Input: part model. Units: mm. Frame: model coordinates. A direction names the side the tool comes from. Give positions to 0.01 mm unless a question says otherwise; leave off trailing zeros. Order: outer loops, then holes, each group sorted by start corner. A loop starts at its lowest first (then second) coordinate and runs counter-clockwise, first axis right, second up. Notation, with made-up numbers: (-3.75, 12.5) - (49.25, 12.5) arc R15 cw to (49.25, 38.5) - close; hole circle Ø1 at (-36, 73). An arc over 180 degrees is marked (long way). Use a Markdown table: item, result.
from build123d import *

# Parameters (mm, degrees)
PAD_DEPTH    = 35
POCKET_DEPTH = 30
SKETCH003_W  = 25
SKETCH003_H  = 15
PAD001_DEPTH = 2
FILLET_R     = 0.99
FILLET001_R  = 0.96
FILLET002_R  = 3


with BuildPart() as part:
    # Sketch → Pad (new body)
    with BuildSketch(Plane.XY):
        with BuildLine():
            ThreePointArc((20, 0), (0, 6.835898), (-20, 0))
            Line((-20, -5.3), (-20, 0))
            Line((20, -5.3), (-20, -5.3))
            Line((20, 0), (20, -5.3))
        make_face()
    extrude(amount=PAD_DEPTH)

    # Sketch002 → Pocket (cut)
    with BuildSketch(Plane(origin=(3, 0, 37), x_dir=(0.965926, 0, -0.258819), z_dir=(0.258819, 0, 0.965926))):
        Polygon((-5.6, -0.240433), (5.6, -0.240433), (5.6, -2.440433), (2.7, -5.340433), (-2.7, -5.340433), (-5.6, -2.440433), align=None)
    extrude(amount=-POCKET_DEPTH, mode=Mode.SUBTRACT)

    # Sketch003 (on Face4 of Pocket) → Pad001 (join)
    with BuildSketch(Plane(origin=(0, 0, 0), x_dir=(1, 0, 0), z_dir=(0, 0, -1))):
        with Locations((0, -10.470599)):
            Rectangle(SKETCH003_W, SKETCH003_H)
    extrude(amount=-PAD001_DEPTH)

    # Fillet
    fillet_edges = [part.edges().sort_by_distance(p)[0] for p in [
        (-12.5, 11.160507, 2),
        (0, 17.970599, 2),
        (12.5, 11.160507, 2),
        (-12.5, 11.160507, 0),
        (0, 17.970599, 0),
        (12.5, 11.160507, 0),
    ]]
    fillet(fillet_edges, radius=FILLET_R)

    # Fillet001
    fillet001_edges = [part.edges().sort_by_distance(p)[0] for p in [
        (-12.149588, 17.620187, 1.765663),
        (-12.149588, 17.620187, 0.234337),
        (12.149588, 17.620187, 0.234337),
        (12.149588, 17.620187, 1.765663),
    ]]
    fillet(fillet001_edges, radius=FILLET001_R)

    # Fillet002
    fillet002_edges = [part.edges().sort_by_distance(p)[0] for p in [
        (-20, 0, 17.5),
        (20, 0, 17.5),
    ]]
    fillet(fillet002_edges, radius=FILLET002_R)


solid = part.part
1. Pin query (flat end, axial travel): pin 1 (2 mm diameter, centred on x = 4, y = 11.5, fed in from +Z); pin 2 (8 mm diameter, centred on y = 4, z = 19.5, fed in from +X); pin 3 (10 mm diameter, centred on y = 5, z = 21.5, fed in from -X); pin 4 (1.5 mm diameter, centred on y = -1, z = 3.5, fed in from +X). Return the tip coordinate at first contact, or that it passes through.
Response:
| item | result |
|---|---|
| pin 1 | stops at z = 2 |
| pin 2 | stops at x = 19.59 |
| pin 3 | stops at x = -19.59 |
| pin 4 | stops at x = 20 |
2. Material intervals for line 1 along Z through (x, y) = (6, 8.5); line 2 along Y through (x, z) = (1.5, 14); line 3 along Y through (x, z) = (-0.5, 9), sorted ascending.
Response:
| item | result |
|---|---|
| line 1 | z = 0 to 2 |
| line 2 | y = -5.3 to -3.54, -0.24 to 6.8 |
| line 3 | y = -5.3 to -4.17, -0.24 to 6.83 |
3. Set-up query: faces 1 (the face through (-12.22, 10.59, 0.3)), 2 (the face through (-4.689, -2.735, 8.002)), 3 (the face through (12.2, 10.59, 1.72)), 4 (the face through (0.16, 17.67, 0.28)). Return all of +Z, -Z, +X, -X, +Y, -Y with unobstructed straight access to the full face (end or side cutting, diameter ignored); none if empty.
Response:
| item | result |
|---|---|
| face 1 | -Z, -X, +Y |
| face 2 | none |
| face 3 | +Z, +X, +Y |
| face 4 | -Z, +X, -X, +Y |
4. Section query A-A (z = 3). Return loops of the section in (x, y).
Response:
| item | result |
|---|---|
| outline | (-20, -5.3) - (20, -5.3) - (20, -1.52) arc R3 ccw to (18.72, 0.94) arc R32.68 ccw to (-18.72, 0.94) arc R3 ccw to (-20, -1.52) - close |
5. Mould query, pull axis Z, two halves, no side actions, for faces 5 (the face through (-5.2, -3.9, 22.4)), 6 (the face through (12.2, 10.59, 0.28)), 7 (the face through (-12.22, 10.59, 1.7)). Classes: pulls with the +Z half, pulls with the -Z half, needs draft (parallel to the pull), parting line crosses it, or undercut.
Response:
| item | result |
|---|---|
| face 5 | undercut |
| face 6 | pulls with the -Z half |
| face 7 | pulls with the +Z half |
